from build123d import *

# Parameters (mm, degrees)
F1_DEPTH = 14
F2_W     = 127
F2_H     = 85
F2_W_2   = 180
F2_H_2   = 22
F2_W_3   = 19
F2_H_3   = 60
F3_DEPTH = 25
F4_R     = 12.5
F5_DEPTH = 25


with BuildPart() as f1:
    # F0 (on Top) → F1 (new body)
    with BuildSketch(Plane.XY):
        with BuildLine():
            ThreePointArc((-135, -87.75), (-131.485281, -96.235281), (-123, -99.75))
            Line((-123, -99.75), (123, -99.75))
            ThreePointArc((123, -99.75), (131.485281, -96.235281), (135, -87.75))
            Line((135, -87.75), (135, 81.331121))
            ThreePointArc((135, 81.331121), (132.403394, 88.429218), (125.839459, 92.17623))
            ThreePointArc((125.839459, 92.17623), (99.105981, 96.217898), (72.244569, 99.296609))
            ThreePointArc((72.244569, 99.296609), (67.790252, 98.888715), (63.794752, 96.877918))
            ThreePointArc((63.794752, 96.877918), (33.680622, 80.80401), (0, 75.25))
            ThreePointArc((0, 75.25), (-33.680622, 80.80401), (-63.794752, 96.877918))
            ThreePointArc((-63.794752, 96.877918), (-67.790252, 98.888715), (-72.244569, 99.296609))
            ThreePointArc((-72.244569, 99.296609), (-99.105981, 96.217898), (-125.839459, 92.17623))
            ThreePointArc((-125.839459, 92.17623), (-132.403394, 88.429218), (-135, 81.331121))
            Line((-135, 81.331121), (-135, -87.75))
        make_face()
    extrude(amount=F1_DEPTH)

    # F2 (on face) → F3 (cut)
    with BuildSketch(Plane.XY.offset(14)):
        with Locations((-26.5, 4.75)):
            Rectangle(F2_W, F2_H)
        with Locations((0, -68.75)):
            Rectangle(F2_W_2, F2_H_2)
        with Locations((80.5, 4.75)):
            Rectangle(F2_W_3, F2_H_3)
    extrude(amount=-F3_DEPTH, mode=Mode.SUBTRACT)

    # F4 (on face) → F5 (cut)
    with BuildSketch(Plane.XY.offset(14)):
        with Locations((-90, 4.75)):
            Circle(F4_R)
        with Locations((90, 4.75)):
            Circle(F4_R)
    extrude(amount=-F5_DEPTH, mode=Mode.SUBTRACT)


solid = f1.part
Check sheet for the modelled part. Datum: model origin and axes. Units: mm. A direction names the side the tool comes from. Coordinates: 2 decimals unless noted, no trailing zeros. Loops run counter-clockwise (first coordinate to the right, second up) from the corner with the lowest first, then second, coordinate; pieces in that order, holes last. Notation, with made-up numbers: (-21.75, 10) -> (33.25, 10) arc R13 ccw to (33.25, 17) -> close; hole circle Ø6 at (3.25, 51.25). An arc over 180 degrees is marked (long way). Write item = value, one per line. Start each with the question number.
1. Material ranges on line 1 (X direction, y = 24.5, z = 13.25); line 2 (Y direction, x = -2.5, z = 5); line 3 (X direction, y = 6, z = 9.5), recorded low to high.
2. Section check B-B on x = -56. Record the cut outline in (y, z).
3. Section check D-D on x = -94.5. Record the cut outline in (y, z).
4. Section check A-A on y = 4.75. Record the cut outline in (x, z).
5. Section check C-C on z = 6. Give the number of separate pieces and of enclosed holes in the cut face, then the cut area to 3 significant figures.
6. Tool access check on faces 1 (the cylindrical face through (-131.58, -96.14, 6.9)), 2 (the flat face through (90, -17, 7)). Record the directions out of +Z, -Z, +X, -X, +Y, -Y that give a thin tool (end or side, any length) a straight path to the whole face; none if there is none.
7. Draft check along X on faces 3 (the flat face through (-2, -43, 14)), 4 (the cylindrical face through (-102.497, 5.025, 7.098)), 5 (the cylindrical face through (-98.731, 96.268, 6.902)). Enter one of: released by +X, released by -X, zero draft, split by the parting line, or undercut.
8. Depth check by flat-ended pin: P1, Ø8, axis at x = 56.5, y = -76, coming from the +Z side; P2, Ø4, axis at x = 79.5, z = 4, coming from the +Y side. Enter the tip coordinate at first touch or a pass-through.
Responses:
q1.line_1 = -135 to -90, 37 to 71, 90 to 135
q1.line_2 = -99.75 to -79.75, -57.75 to -37.75, 47.25 to 75.28
q1.line_3 = -135 to -102.44, 37 to 71, 102.44 to 135
q2.outline = (-99.75, 0) -> (-79.75, 0) -> (-79.75, 14) -> (-99.75, 14) -> close; (-57.75, 0) -> (-37.75, 0) -> (-37.75, 14) -> (-57.75, 14) -> close; (47.25, 0) -> (91.45, 0) -> (91.45, 14) -> (47.25, 14) -> close
q3.outline = (-99.75, 0) -> (-6.91, 0) -> (-6.91, 14) -> (-99.75, 14) -> close; (16.41, 0) -> (96.82, 0) -> (96.82, 14) -> (16.41, 14) -> close
q4.outline = (-135, 0) -> (-102.5, 0) -> (-102.5, 14) -> (-135, 14) -> close; (37, 0) -> (71, 0) -> (71, 14) -> (37, 14) -> close; (102.5, 0) -> (135, 0) -> (135, 14) -> (102.5, 14) -> close
q5.separate_pieces = 1
q5.enclosed_holes = 3
q5.area = 34,600 mm2
q6.face_1 = +Z, -Z, -X, -Y
q6.face_2 = +Z, -Z
q7.face_3 = zero draft
q7.face_4 = undercut
q7.face_5 = released by -X
q8.P1 = 14
q8.P2 = 98.77
